```python
from build123d import *

# Parameters (mm, degrees)
F0_W     = 196.85
F0_H     = 25.4
F1_DEPTH = 25.4
F2_R     = 12.7
F4_DEPTH = 25.4
F5_D     = 6.5278
F7_D     = 6.5278


with BuildPart() as f1:
    # F0 (on Front) → F1 (new body)
    with BuildSketch(Plane.XZ):
        with Locations((98.425, 12.7)):
            Rectangle(F0_W, F0_H)
    extrude(amount=F1_DEPTH)

    # F2 (on face) → F4 (cut)
    with BuildSketch(Plane.XZ.offset(25.4)):
        with Locations((38.1, 0)):
            Circle(F2_R)
    extrude(amount=-F4_DEPTH, mode=Mode.SUBTRACT)

    # F5 (through all)
    with Locations(Plane.XZ.offset(25.4)):
        with Locations((157.1625, 12.7), (182.5625, 12.7)):
            Hole(F5_D / 2)

    # F7 (through all)
    with Locations(Plane(origin=(0, 0, 0), x_dir=(1, 0, 0), z_dir=(0, 0, -1))):
        with Locations((12.7, 12.7), (63.5, 12.7)):
            Hole(F7_D / 2)


solid = f1.part
```
Part model, mm, in its own coordinate system. Round coordinates to 2 decimals unless told otherwise and drop trailing zeros. Loops run counter-clockwise (first coordinate to the right, second up) from the corner with the lowest first, then second, coordinate; pieces in that order, holes last. Notation, with made-up numbers: (-25, 7.25) -> (25, 7.25) arc R21 ccw to (25, 35.25) -> close; hole circle Ø1 at (58, -7). An arc over 180 degrees is marked (long way). Use a Markdown table: item, result.
1) Pull direction X, two halves, no side cores. Call faces 1 (the cylindrical face through (64.208, -9.514, 12.878)), 2 (the flat face through (196.85, -13, 13)), 3 (the flat face through (123, -13, 0)), 4 (the cylindrical face through (160.423, -12.522, 12.844)): pulls with the +X half, pulls with the -X half, needs draft (parallel to the pull), parting line crosses it, or undercut.
The answers:
| item | result |
|---|---|
| face 1 | undercut |
| face 2 | pulls with the +X half |
| face 3 | needs draft |
| face 4 | undercut |
2) Cut at B-B, the plane x = 12.7. List the corners of the cut face in (y, z), and give its area (3 significant figures).
The answers:
| item | result |
|---|---|
| outline | (-25.4, 0) -> (-15.96, 0) -> (-15.96, 25.4) -> (-25.4, 25.4) -> close; (-9.44, 0) -> (0, 0) -> (0, 25.4) -> (-9.44, 25.4) -> close |
| area | 479 mm2 |
3) Probe line 1 (Y direction, x = 12.7, z = 20); line 2 (X direction, y = -11.5, z = 7); line 3 (X direction, y = -12, z = 6.5). List the from-to ranges inside material, lowest first. Write a range as [from, to].
The answers:
| item | result |
|---|---|
| line 1 | y = [-25.4, -15.96], [-9.44, 0] |
| line 2 | x = [0, 9.66], [15.74, 27.5], [48.7, 60.46], [66.54, 196.85] |
| line 3 | x = [0, 9.51], [15.89, 27.19], [49.01, 60.31], [66.69, 196.85] |
4) Cut at D-D, the plane z = 4.5. List the corners of the cut face in (x, y), and give its area (3 significant figures).
The answers:
| item | result |
|---|---|
| outline | (0, -25.4) -> (26.22, -25.4) -> (26.22, 0) -> (0, 0) -> close; (49.98, -25.4) -> (196.85, -25.4) -> (196.85, 0) -> (49.98, 0) -> close; hole circle Ø6.53 at (12.7, -12.7); hole circle Ø6.53 at (63.5, -12.7) |
| area | 4,330 mm2 |
5) Cut at C-C, the plane y = -5. List the corners of the cut face in (x, z).
The answers:
| item | result |
|---|---|
| outline | (0, 0) -> (25.4, 0) arc R12.7 cw to (50.8, 0) -> (196.85, 0) -> (196.85, 25.4) -> (0, 25.4) -> close; hole circle Ø6.53 at (157.16, 12.7); hole circle Ø6.53 at (182.56, 12.7) |
6) Cut at A-A, the plane y = -12.7. List the corners of the cut face in (x, z), and give its area (3 significant figures).
The answers:
| item | result |
|---|---|
| outline | (0, 0) -> (9.44, 0) -> (9.44, 25.4) -> (0, 25.4) -> close; (15.96, 0) -> (25.4, 0) arc R12.7 cw to (50.8, 0) -> (60.24, 0) -> (60.24, 25.4) -> (15.96, 25.4) -> close; (66.76, 0) -> (196.85, 0) -> (196.85, 25.4) -> (66.76, 25.4) -> close; hole circle Ø6.53 at (157.16, 12.7); hole circle Ø6.53 at (182.56, 12.7) |
| area | 4,350 mm2 |
7) Drop a flat-ended pin along its axis: pin 1 Ø6 at (x, y) = (12.7, -12.7) entering from +Z. Give the stop position or say it passes through.
The answers:
| item | result |
|---|---|
| pin 1 | passes through |
